```python
from build123d import *

# Parameters (mm, degrees)
SALIENTE_EXTRUIR1_DEPTH = 5
CROQUIS2_R              = 2
SALIENTE_EXTRUIR2_DEPTH = 5


with BuildPart() as part:
    # Croquis1 → Saliente-Extruir1 (new body)
    with BuildSketch(Plane.XY):
        with BuildLine():
            Line((-25.953664325, 5.804713338), (22.678050908, 5.804713338))
            ThreePointArc((22.678050908, 5.804713338), (27.678050908, 0.804713338), (22.678050908, -4.195286662))
            Line((22.678050908, -4.195286662), (-23.047151147, -4.195286662))
            ThreePointArc((-23.047151147, -4.195286662), (-41.661617991, 4.287687085), (-51.741257509, 22.088251307))
            ThreePointArc((-51.741257509, 22.088251307), (-48.695784379, 32.499543684), (-42.578743977, 23.541210565))
            ThreePointArc((-42.578743977, 23.541210565), (-36.695300038, 12.396079877), (-25.953664325, 5.804713338))
        make_face()
    extrude(amount=SALIENTE_EXTRUIR1_DEPTH)

    # Croquis2 → Saliente-Extruir2 (add)
    with BuildSketch(Plane.XY.offset(5)):
        with Locations((22.678050908, 0.804713338)):
            Circle(CROQUIS2_R)
    extrude(amount=SALIENTE_EXTRUIR2_DEPTH)


solid = part.part
```
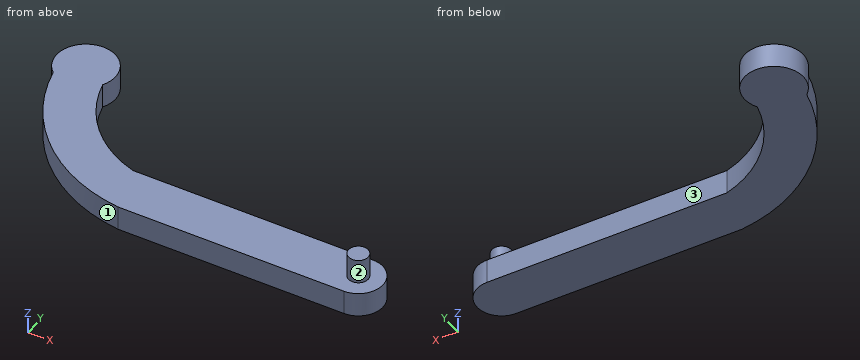
For this review, take the finished solid that the model builds, in its own axes (mm). Face numbers are marked on the shaded views. A direction names the side the tool comes from. Give positions to 0.01 mm unless a question says otherwise; leave off trailing zeros. Write each loop counter-clockwise with the first axis right and the second up, starting at its lowest first coordinate (ties: lowest second). Pieces come first, ordered by that corner, then holes.
Item 1: Machinability: for the marked faces 1, 2 and 3, which of the approach directions +Z, -Z, +X, -X, +Y, -Y give a long, thin tool a straight path to every point of the face, cutting with its end or side? Answer none if there is none.
Item 2: Take a section at C-C (y = 0). Give the boundary of the cut face in (x, z), and give its area (3 significant figures).
Item 3: Take a section at D-D (y = 21). Give the boundary of the cut face in (x, z), and give its area (3 significant figures).
Item 4: Insertion check: P1, Ø10, axis at x = -0.5, y = 6, coming from the -Z side; P2, Ø1, axis at y = 0, z = 9, coming from the -X side; P3, Ø1.5, axis at x = 17, z = 2, coming from the +Y side; P4, Ø10, axis at x = -28.5, y = 12, coming from the +Z side. Each pin has a flat end and moves straight along its axis. Give the tip position at first contact, or say it passes through.
Item 5: Wall thickness on probe 1 along Y at (x, z) = (-21.5, 1.75); probe 2 along Z at (x, y) = (-46, 28.5); probe 3 along X at (y, z) = (-1, 5.5): over which ranges is each line inside the solid? List them lowest first.
Item 6: Take a section at A-A (z = 3.25). Give the boundary of the cut face in (x, y).
Item 7: Take a section at B-B (x = 10.5). Give the boundary of the cut face in (y, z), and give its area (3 significant figures).
Established:
1. face 1: +Z, -Z, -X, -Y
1. face 2: +Z
1. face 3: +Z, -Z, +X, +Y
2. outline: (-35.8, 0) - (27.61, 0) - (27.61, 5) - (24.51, 5) - (24.51, 10) - (20.85, 10) - (20.85, 5) - (-35.8, 5) - close
2. area: 335 mm2
3. outline: (-51.5, 0) - (-41.87, 0) - (-41.87, 5) - (-51.5, 5) - close
3. area: 48.2 mm2
4. P1: stops at z = 0
4. P2: stops at x = 20.7
4. P3: stops at y = 5.8
4. P4: stops at z = 5
5. probe 1: y = -4.2 to 5.8
5. probe 2: z = 0 to 5
5. probe 3: x = 21.82 to 23.54
6. outline: (-51.74, 22.09) arc R33.12 ccw to (-23.05, -4.2) - (22.68, -4.2) arc R5 ccw to (22.68, 5.8) - (-25.95, 5.8) arc R23.85 cw to (-42.58, 23.54) arc R6 ccw (long way) to start
7. outline: (-4.2, 0) - (5.8, 0) - (5.8, 5) - (-4.2, 5) - close
7. area: 50.0 mm2
